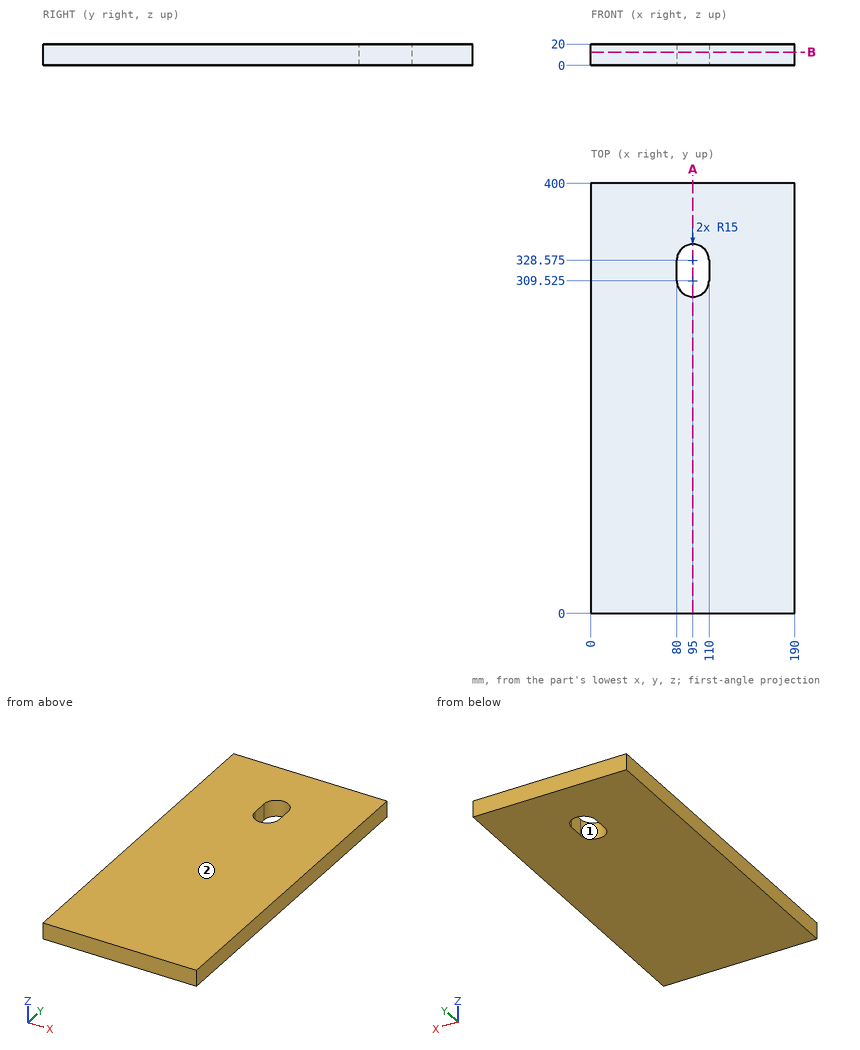
Geometry: see drawing. Coordinates: mm, zero at the bounding-box minimum. Give positions to 0.01 mm unless a question says otherwise; leave off trailing zeros. Order: outer loops, then holes, each group sorted by start corner. A loop starts at its lowest first (then second) coordinate and runs counter-clockwise, first axis right, second up.
1. Pin query (flat end, axial travel): pin 1 Ø5 at (x, z) = (67.5, 8) entering from -Y. Return the tip coordinate at first contact, or that it passes through.
Computed:
pin 1: stops at y = 0
2. Cut plane A-A (x = 95). Return loops of the section in (y, z) (3 decimals), and give its area (3 significant figures).
Computed:
outline: (0, 0) - (294.525, 0) - (294.525, 20) - (0, 20) - close; (343.575, 0) - (400, 0) - (400, 20) - (343.575, 20) - close
area: 7,020 mm2
3. Cut plane B-B (z = 12.5). Return loops of the section in (x, y) (3 decimals).
Computed:
outline: (0, 0) - (190, 0) - (190, 400) - (0, 400) - close; hole (80, 309.525) arc R15 ccw to (110, 309.525) - (110, 328.575) arc R15 ccw to (80, 328.575) - close
4. Line query: probe 1 along X at (y, z) = (342.5, 13.5); probe 2 along Y at (x, z) = (84.5, 16.25); probe 3 along X at (y, z) = (332, 3.25). Output: solid intervals per line, ascending.
Computed:
probe 1: x = 0 to 89.42, 100.58 to 190
probe 2: y = 0 to 298.81, 339.29 to 400
probe 3: x = 0 to 80.4, 109.6 to 190
5. Draft query along X for the marked faces 1 and 2. Return one class per face: released by +X, released by -X, zero draft, split by the parting line, or undercut.
Computed:
face 1: undercut
face 2: zero draft
